The model under review builds one solid part; all positions refer to its coordinate system, in mm. Give positions to 0.01 mm unless a question says otherwise; leave off trailing zeros. Order: outer loops, then holes, each group sorted by start corner. A loop starts at its lowest first (then second) coordinate and runs counter-clockwise, first axis right, second up. Notation, with made-up numbers: (-14, -27) - (24, -27) arc R8 ccw to (24, -22) - close; hole circle Ø6 at (69.25, 40). An arc over 180 degrees is marked (long way). Use a Markdown table: item, result. Add a question column.
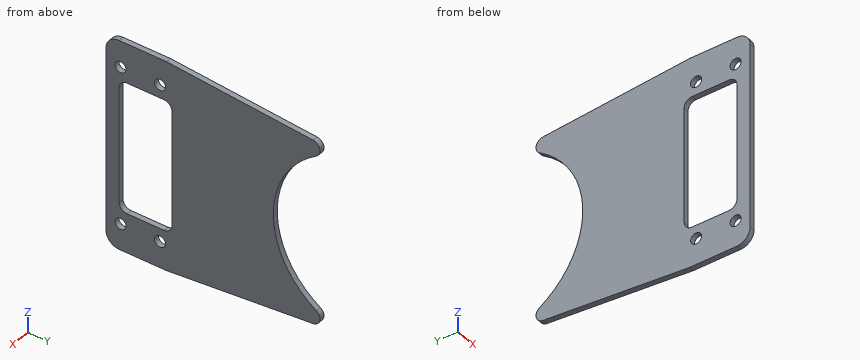
```python
from build123d import *

# Parameters (mm, degrees)
EXTRUDE_1_DEPTH     = 2
SKETCH_2_R          = 2.1
SKETCH_2_W          = 50
SKETCH_2_H          = 20
CUT_EXTRUDE_1_DEPTH = 2
FILLET_1_R          = 3
FILLET_2_R          = 5


with BuildPart() as part:
    # 草图1 → 凸台-拉伸1 (new body)
    with BuildSketch(Plane(origin=(0, 0, 0), x_dir=(0, 0, -1), z_dir=(1, 0, 0))):
        with BuildLine():
            Line((-40, 11.5), (-34.088778562, 79.065570207))
            ThreePointArc((-34.088778562, 79.065570207), (0, 52), (34.088778562, 79.065570207))
            Line((34.088778562, 79.065570207), (40, 11.5))
            Line((40, 11.5), (40, -11.5))
            Line((40, -11.5), (-40, -11.5))
            Line((-40, -11.5), (-40, 11.5))
        make_face()
    extrude(amount=EXTRUDE_1_DEPTH)

    # 草图2 → 切除-拉伸1 (cut)
    with BuildSketch(Plane(origin=(2, 0, 0), x_dir=(0, 0, -1), z_dir=(1, 0, 0))):
        with Locations((-30, 9)):
            Circle(SKETCH_2_R)
        with Locations((-30, -6)):
            Circle(SKETCH_2_R)
        with Locations((30, -6)):
            Circle(SKETCH_2_R)
        with Locations((30, 9)):
            Circle(SKETCH_2_R)
        with Locations((0, 3.5)):
            Rectangle(SKETCH_2_W, SKETCH_2_H)
    extrude(amount=-CUT_EXTRUDE_1_DEPTH, mode=Mode.SUBTRACT)

    # 圆角1
    fillet_1_edges = [part.edges().sort_by_distance(p)[0] for p in [
        (1, 79.065570207, 34.088778562),
        (1, 79.065570207, -34.088778562),
        (1, 13.5, -25),
        (1, -6.5, -25),
        (1, -6.5, 25),
        (1, 13.5, 25),
    ]]
    fillet(fillet_1_edges, radius=FILLET_1_R)

    # 圆角2
    fillet_2_edges = [part.edges().sort_by_distance(p)[0] for p in [
        (1, -11.5, -40),
        (1, -11.5, 40),
    ]]
    fillet(fillet_2_edges, radius=FILLET_2_R)


solid = part.part
```
Q1. We need section B-B (z = -20.5). Write out the cut boundary in (x, y), plus the area to 3 significant figures.
Q2. We need section A-A (y = 9). Write out the cut boundary in (x, z), plus the area to 3 significant figures.
Q3. Wall thickness on probe 1 along Y at (x, z) = (0.7, 30); probe 2 along Z at (x, y) = (1.85, -3.5); probe 3 along Y at (x, z) = (1.3, -29): over which ranges is each line inside the solid? List them lowest first.
Q4. We need section C-C (x = 0.3). Write out the cut boundary in (y, z), plus the area to 3 significant figures.
Q5. We need section D-D (y = 63). Write out the cut boundary in (x, z), plus the area to 3 significant figures.
Here are the results:
| question | item | result |
|---|---|---|
| 1 | outline | (0, -11.5) - (2, -11.5) - (2, -6.5) - (0, -6.5) - close; (0, 13.5) - (2, 13.5) - (2, 58.63) - (0, 58.63) - close |
| 1 | area | 100 mm2 |
| 2 | outline | (0, -40) - (2, -40) - (2, -32.1) - (0, -32.1) - close; (0, -27.9) - (2, -27.9) - (2, -25) - (0, -25) - close; (0, 25) - (2, 25) - (2, 27.9) - (0, 27.9) - close; (0, 32.1) - (2, 32.1) - (2, 40) - (0, 40) - close |
| 2 | area | 43.2 mm2 |
| 3 | probe 1 | -11.5 to -8.1, -3.9 to 6.9, 11.1 to 68.84 |
| 3 | probe 2 | -40 to -25, 25 to 40 |
| 3 | probe 3 | -11.5 to -7.85, -4.15 to 7.15, 10.85 to 67.4 |
| 4 | outline | (-11.5, -35) arc R5 ccw to (-6.5, -40) - (11.5, -40) - (67.01, -35.14) arc R3 ccw to (68.35, -29.62) arc R35 cw to (68.35, 29.62) arc R3 ccw to (67.01, 35.14) - (11.5, 40) - (-6.5, 40) arc R5 ccw to (-11.5, 35) - close; hole circle Ø4.2 at (-6, -30); hole circle Ø4.2 at (-6, 30); hole (-6.5, -22) arc R3 ccw to (-3.5, -25) - (10.5, -25) arc R3 ccw to (13.5, -22) - (13.5, 22) arc R3 ccw to (10.5, 25) - (-3.5, 25) arc R3 ccw to (-6.5, 22) - close; hole circle Ø4.2 at (9, -30); hole circle Ø4.2 at (9, 30) |
| 4 | area | 4,370 mm2 |
| 5 | outline | (0, -35.49) - (2, -35.49) - (2, -25.48) - (0, -25.48) - close; (0, 25.48) - (2, 25.48) - (2, 35.49) - (0, 35.49) - close |
| 5 | area | 40.1 mm2 |
